```python
from build123d import *

# Parameters (mm, degrees)
SKETCH1_W           = 50.8
SKETCH1_H           = 50.8
BOSS_EXTRUDE1_DEPTH = 50.8
SKETCH2_W           = 12.8016
SKETCH2_H           = 12.71524
SKETCH2_W_2         = 26.9875
SKETCH2_H_2         = 25.36952
CUT_EXTRUDE1_DEPTH  = 108.763073453
SKETCH3_W           = 3.96875
SKETCH3_H           = 23.8125
BOSS_EXTRUDE2_DEPTH = 50.00625
SKETCH4_R           = 11.90625
BOSS_EXTRUDE3_DEPTH = 25.4
SKETCH5_W           = 50.8
SKETCH5_H           = 15.875
BOSS_EXTRUDE4_DEPTH = 19.05
SKETCH6_W           = 7.9375
SKETCH6_H           = 7.9375
BOSS_EXTRUDE5_DEPTH = 12.7
FILLET1_R           = 0.762


with BuildPart() as part:
    # Sketch1 → Boss-Extrude1 (new, symmetric)
    with BuildSketch(Plane(origin=(0, 0, 0), x_dir=(0, 0, -1), z_dir=(1, 0, 0))):
        Rectangle(SKETCH1_W, SKETCH1_H)
    extrude(amount=BOSS_EXTRUDE1_DEPTH, both=True)

    # Sketch2 → Cut-Extrude1 (cut, through all)
    with BuildSketch(Plane(origin=(50.8, 0, 0), x_dir=(0, 0, -1), z_dir=(1, 0, 0))):
        with Locations((0, 19.04238)):
            Rectangle(SKETCH2_W, SKETCH2_H)
        Rectangle(SKETCH2_W_2, SKETCH2_H_2)
    extrude(amount=-CUT_EXTRUDE1_DEPTH, mode=Mode.SUBTRACT)

    # Sketch3 → Boss-Extrude2 (add)
    with BuildSketch(Plane.XZ.offset(25.4)):
        Rectangle(SKETCH3_W, SKETCH3_H)
    extrude(amount=BOSS_EXTRUDE2_DEPTH)

    # Sketch4 → Boss-Extrude3 (add, symmetric)
    with BuildSketch(Plane.XY):
        with Locations((0, -75.40625)):
            Circle(SKETCH4_R)
    extrude(amount=BOSS_EXTRUDE3_DEPTH, both=True)

    # Sketch5 → Boss-Extrude4 (add)
    with BuildSketch(Plane.ZY.offset(50.8)):
        with Locations((0, -17.4625)):
            Rectangle(SKETCH5_W, SKETCH5_H)
    extrude(amount=BOSS_EXTRUDE4_DEPTH)

    # Sketch6 → Boss-Extrude5 (add)
    with BuildSketch(Plane.XZ.offset(25.4)):
        with Locations((39.53002, 0)):
            Rectangle(SKETCH6_W, SKETCH6_H)
    extrude(amount=BOSS_EXTRUDE5_DEPTH)

    # Fillet1
    fillet1_edges = [part.edges().sort_by_distance(p)[0] for p in [
        (-50.8, -12.68476, 0),
        (1.984375, -63.66652918, 0),
        (-1.984375, -63.66652918, 0),
    ]]
    fillet(fillet1_edges, radius=FILLET1_R)


solid = part.part
```
Design review of the part built by this model. Coordinates are the model's own, in mm. A direction names the side the tool comes from. Give positions to 0.01 mm unless a question says otherwise; leave off trailing zeros. Order: outer loops, then holes, each group sorted by start corner. A loop starts at its lowest first (then second) coordinate and runs counter-clockwise, first axis right, second up. Notation, with made-up numbers: (41, 88) -> (79, 88) arc R18 cw to (79, 96) -> close; hole circle Ø3 at (52.25, 84). An arc over 180 degrees is marked (long way). Write item = value, one per line. Start each with the question number.
(1) To check wall thickness, follow line 1 along Y through (x, z) = (7.5, 6.5); line 2 along Y through (x, z) = (-42.5, 8); line 3 along X through (y, z) = (19.5, -7). State the ranges of each line that lie inside material, in increasing order.
(2) For pin 1 (6 mm diameter, centred on x = -5.5, z = -8.5, fed in from -Y); pin 2 (1 mm diameter, centred on x = 27.5, z = -17, fed in from -Y); pin 3 (4 mm diameter, centred on x = 0.5, y = -43, fed in from +Z); pin 4 (12 mm diameter, centred on x = 38, z = 3.5, fed in from +Y), all flat-tipped, find the tip position at first contact; note any pin that passes through.
(3) Mouldability with a two-part tool opening along Y and no side actions: class faces 1 (the face through (39, -38.1, 0)), 2 (the face through (1.984, -44, 0)), 3 (the face through (-9, 0, 25.4)) as +Y half, -Y half, draft (parallel to the pull), parting line (faces both ways), or undercut.
(4) For faces 4 (the face through (43.499, -32, 0)), 5 (the face through (-50.8, 8, 18)), 6 (the face through (39, -32, -3.969)), 7 (the face through (1, 19, 6.401)), 8 (the face through (35.561, -32, 0)), list the 3-axis set-ups (+Z, -Z, +X, -X, +Y, -Y) from which the entire face can be reached by the end or side of a thin tool; tool diameter is ignored.
(5) We need section B-B on x = -44.5. Write out the cut boundary in (y, z), plus the area to 3 significant figures.
Numbers:
q1.line_1 = -84.65 to -66.16, -25.4 to -12.68, 12.68 to 25.4
q1.line_2 = -25.4 to -12.68, 12.68 to 25.4
q1.line_3 = -50.8 to 50.8
q2.pin_1 = -87.05
q2.pin_2 = -25.4
q2.pin_3 = 11.91
q2.pin_4 = 25.4
q3.face_1 = -Y half
q3.face_2 = undercut
q3.face_3 = draft
q4.face_4 = +Z, -Z, +X, -Y
q4.face_5 = +Z, -Z, -X, +Y
q4.face_6 = -Z, +X, -Y
q4.face_7 = +X, -X, +Y
q4.face_8 = +Z, -Z, -Y
q5.outline = (-25.4, -25.4) -> (25.4, -25.4) -> (25.4, -6.4) -> (12.68, -6.4) -> (12.68, -13.49) -> (-12.68, -13.49) -> (-12.68, 13.49) -> (12.68, 13.49) -> (12.68, 6.4) -> (25.4, 6.4) -> (25.4, 25.4) -> (-25.4, 25.4) -> close
q5.area = 1,730 mm^2
